Check sheet for the modelled part. Datum: model origin and axes. Units: mm. A direction names the side the tool comes from. Coordinates: 2 decimals unless noted, no trailing zeros. Loops run counter-clockwise (first coordinate to the right, second up) from the corner with the lowest first, then second, coordinate; pieces in that order, holes last.
Autodesk Inventor part; units mm, degrees
ref_plane "YZ Plane" through (0, 0, 0) normal (1, 0, 0) x (0, 1, 0)
ref_plane "XZ Plane" through (0, 0, 0) normal (0, 1, 0) x (-1, 0, 0)
ref_plane "XY Plane" through (0, 0, 0) normal (0, 0, 1) x (1, 0, 0)
sketch "Sketch1" plane through (0, 0, 0) normal (0, 1, 0) x (-1, 0, 0)
  circle A0 centre (0, 0) radius 105
  dimension "d0" = 210
extrude "Extrusion1" add sketch "Sketch1" along normal blind 10
sketch "Sketch2" plane through (0, 10, 0) normal (0, 1, 0) x (1, 0, 0)
  line L0 (-79.8594, -68.6516) -> (79.5179, -68.6516)
  line L1 (0, 0) -> (0, -80)
  line L2 (0, -80) -> (0, -60)
  line L3 (0, -60) -> (17.5, -60)
  line L4 (0, -60) -> (-17.5, -60)
  circle A0 centre (-17.5, -60) radius 2.5
  circle A1 centre (0, -60) radius 2.5
  circle A2 centre (17.5, -60) radius 2.5
  dimension "d4" = 80
  dimension "d5" = 20
  dimension "d6" = 17.5
  dimension "d7" = 17.5
  dimension "d8" = 5
  dimension "d9" = 5
  dimension "d10" = 5
extrude "Extrusion2" cut sketch "Sketch2" against normal blind 10
sketch "Sketch3" plane through (0, 10, 0) normal (0, 1, 0) x (1, 0, 0)
  circle A0 centre (0, 0) radius 2.5
  dimension "d13" = 5
extrude "Extrusion3" cut sketch "Sketch3" against normal blind 10
sketch "Sketch4" plane through (0, 10, 0) normal (0, 1, 0) x (1, 0, 0)
  circle A0 centre (0, 0) radius 2.5
  line L0 (0, 0) -> (0, 80)
  line L1 (-15, 80) -> (-15, 65)
  line L2 (-15, 65) -> (15, 65)
  line L3 (15, 65) -> (15, 95)
  line L4 (15, 95) -> (-15, 95)
  line L5 (-15, 95) -> (-15, 80)
  line L6 (0, 80) -> (-7.5, 80)
  line L7 (-7.5, 80) -> (7.5, 80)
  line L8 (7.5, 80) -> (7.5, 95)
  line L9 (7.5, 80) -> (7.5, 65)
  line L10 (-7.5, 80) -> (-7.5, 95)
  line L11 (-7.5, 80) -> (-7.5, 65)
  dimension "d20" = 15
  dimension "d21" = 15
  dimension "d22" = 30
  dimension "d23" = 30
  dimension "d24" = 7.5
  dimension "d25" = 15
extrude "Extrusion4" add sketch "Sketch4" along normal blind 30 contours L2 L11 L6 L0 | L0 L7 L9 L2 | L6 L10 L4 L8 L7
sketch "Sketch5" plane through (7.5, 10, -65) normal (1, 0, 0) x (0, 0, -1)
  line L0 (40, 0) -> (-170, 0)
  line L1 (40, 0) -> (15, 0)
  line L2 (15, 0) -> (15, 15)
  circle A0 centre (15, 15) radius 7.5
  line L3 (30, 0) -> (30, 30)
  arc A1 (30, 15) -> (0, 15) centre (15, 15) ccw
  line L4 (15, 15) -> (0, 15) construction
  line L5 (15, 15) -> (30, 15) construction
  line L6 (0, 0) -> (0, 30)
  line L7 (0, 15) -> (0, 30)
  line L8 (0, 30) -> (30, 30)
  line L9 (0, 30) -> (30, 30)
  line L10 (30, 30) -> (30, 15)
  point P0 (-65, -10)
  point P1 (15, 30)
  dimension "d28" = 25
  dimension "d29" = 15
  dimension "d30" = 15
  dimension "d31" = 180
extrude "Extrusion5" cut sketch "Sketch5" against normal blind 30 contours A1 L8 L3 | A1 L6 L8 | A0
sketch "Sketch6" plane through (7.5, 10, -65) normal (1, 0, 0) x (0, 0, -1)
  circle A0 centre (15, 15) radius 7.5
  circle A1 centre (15, 15) radius 5
  circle A2 centre (15, 15) radius 7.5
  point P0 (-65, -10)
  dimension "d34" = 10
extrude "Extrusion6" add sketch "Sketch6" against normal blind 15
sketch "Sketch7" plane through (7.5, 10, -65) normal (1, 0, 0) x (0, 0, -1)
  line L0 (0, 0) -> (30, 0)
  line L1 (0, 0) -> (30, 0)
  line L2 (30, 0) -> (30, 34.6991)
  line L3 (30, 34.6991) -> (0, 34.6991)
  line L4 (0, 34.6991) -> (0, 0)
  point P0 (-65, -10)
extrude "Extrusion7" cut sketch "Sketch7" against normal blind 15
sketch "Sketch8" plane through (0, 10, 0) normal (0, 1, 0) x (1, 0, 0)
  circle A0 centre (0, 0) radius 2.5
  line L0 (0, 0) -> (0, 100)
  line L1 (0, 100) -> (-10, 100)
  line L2 (-10, 100) -> (-20, 100)
  line L3 (-20, 100) -> (-20, 65)
  line L4 (-20, 65) -> (-10, 65)
  line L5 (-10, 65) -> (-10, 100)
  line L6 (0, 100) -> (10, 100)
  line L7 (10, 100) -> (20, 100)
  line L8 (20, 100) -> (20, 65)
  line L9 (20, 65) -> (10, 65)
  line L10 (10, 65) -> (10, 100)
  dimension "d42" = 100
  dimension "d43" = 10
  dimension "d44" = 10
  dimension "d45" = 35
  dimension "d46" = 10
  dimension "d47" = 10
  dimension "d48" = 35
extrude "Extrusion8" add sketch "Sketch8" along normal blind 35 contours L5 L4 L3 L2 | L7 L8 L9 L10
thicken "Thicken1" operation add thickness 5 both sides no extend neighbours yes toward (0, 1, 0) faces at (13.3333, 45, -88.3333)
thicken "Thicken2" operation add thickness 5 both sides no extend neighbours yes toward (0, 1, 0) faces at (-16.6667, 45, -88.3333)
sketch "Sketch10" plane through (20, 10, -65) normal (1, 0, 0) x (0, 0, -1)
  line L0 (0, 0) -> (35, 0)
  line L1 (0, 0) -> (17.5, 0)
  line L2 (17.5, 0) -> (17.5, 22.5)
  circle A0 centre (17.5, 22.5) radius 12.5
  circle A1 centre (17.5, 22.5) radius 17.5
  line L3 (35, 0) -> (35, 40)
  line L4 (0, 0) -> (0, 40)
  line L5 (0, 22.5) -> (0, 40)
  line L6 (35, 40) -> (0, 40)
  line L7 (0, 40) -> (35, 40)
  line L8 (35, 40) -> (35, 22.5)
  point P0 (-65, -10)
  point P1 (17.5, 40)
  dimension "d60" = 22.5
  dimension "d61" = 25
extrude "Extrusion9" cut sketch "Sketch10" against normal blind 40 contours L4 L6 A1 | L6 L3 A1 | A0
sketch "Sketch11" plane through (20, 10, -65) normal (1, 0, 0) x (0, 0, -1)
  line L0 (40, 0) -> (-170, 0)
  line L1 (35.2175, 0) -> (0.2175, 0)
  line L2 (0.2175, 0) -> (-34.7825, 0)
  line L3 (0.2175, 0) -> (40.2175, 0)
  circle A0 centre (40.2175, 17.5) radius 12.5
  circle A1 centre (40.2175, 17.5) radius 17.5
  line L4 (-34.7825, 0) -> (32.4725, 33.1928)
  point P0 (-65, -10)
  dimension "d73" = 35
  dimension "d74" = 35
  dimension "d75" = 40
  dimension "d78" = 35
sketch "Sketch12" plane through (-20, 10, -100) normal (-1, 0, 0) x (0, 0, 1)
  line L0 (205, 0) -> (-5, 0)
  line L1 (37.401, 0) -> (37.401, 45.2729)
  line L2 (37.401, 45.2729) -> (-3.1543, 48.8051)
  line L3 (-3.1543, 48.8051) -> (-3.1543, 0)
  line L4 (37.401, 0) -> (-3.1543, 0)
  point P0 (100, -10)
extrude "Extrusion10" cut sketch "Sketch12" against normal blind 40
extrude "Extrusion11" add sketch "Sketch11" against normal blind 40
sketch "Sketch13" plane through (0, 0, 0) normal (0, 0, 1) x (1, 0, 0)
  line L0 (105, 10) -> (-105, 10)
  line L1 (0, 10) -> (10, 10)
  line L2 (10, 10) -> (10, 48.8421)
  line L3 (20, 43.1928) -> (-20, 43.1928)
  line L4 (10, 48.8421) -> (-10, 48.8421)
  line L5 (-10, 48.8421) -> (-10, 10)
  line L6 (-10, 10) -> (10, 10)
  point P0 (0, 0)
  point P1 (-20, 10)
  point P2 (20, 10)
  dimension "d83" = 10
  dimension "d84" = 20
extrude "Extrusion12" cut sketch "Sketch13" against normal blind 150
sketch "Sketch14" plane through (20, 10, -65) normal (1, 0, 0) x (0, 0, -1)
  line L0 (38.0776, 0) -> (-34.7825, 0)
  line L1 (-34.7825, 0) -> (42.8397, 49.7383)
  line L2 (42.8397, 49.7383) -> (77.8644, 0)
  line L3 (77.8644, 0) -> (-34.7825, 0)
  point P0 (-65, -10)
extrude "Extrusion13" cut sketch "Sketch14" against normal blind 150
sketch "Sketch15" plane through (0, 10, 0) normal (0, 1, 0) x (1, 0, 0)
  circle A0 centre (0, 0) radius 2.5
  line L0 (0, 0) -> (0, 100)
  line L1 (0, 100) -> (-20, 100)
  line L2 (-20, 100) -> (-20, 65)
  line L3 (-20, 65) -> (-10, 65)
  line L4 (-10, 65) -> (-10, 100)
  line L5 (-10, 65) -> (10, 65)
  line L6 (10, 65) -> (20, 65)
  line L7 (20, 65) -> (20, 100)
  line L8 (20, 100) -> (10, 100)
  line L9 (10, 100) -> (10, 65)
  dimension "d89" = 100
  dimension "d90" = 20
  dimension "d91" = 35
  dimension "d92" = 10
  dimension "d93" = 20
  dimension "d94" = 10
  dimension "d95" = 35
  dimension "d96" = 10
extrude "Extrusion14" add sketch "Sketch15" along normal blind 40 contours L3 L2 L1 L4 | L9 L8 L7 L6
sketch "Sketch16" plane through (20, 10, -65) normal (1, 0, 0) x (0, 0, -1)
  line L0 (0, 40) -> (35, 40)
  line L1 (17.5, 40) -> (17.5, 22.5)
  circle A0 centre (17.5, 22.5) radius 12.5
  circle A1 centre (17.5, 22.5) radius 17.5
  line L2 (35, 0) -> (35, 40)
  line L3 (0, 0) -> (0, 40)
  line L4 (0, 22.5) -> (0, 40)
  line L5 (0, 40) -> (35, 40)
  line L6 (35, 40) -> (35, 22.5)
  point P0 (-65, -10)
  dimension "d99" = 17.5
  dimension "d100" = 25
extrude "Extrusion15" cut sketch "Sketch16" against normal blind 40 contours L0 A1 L3 | L0 L2 A1 | A0
properties part number "Base do telescópio"
1) Mould release check, pull along Y, two halves, no side actions. Record for faces 4 (the cylindrical face through (-14.93, 49.996, -82.885)), 5 (the cylindrical face through (-14.93, 27.712, -94.047)), 6 (the flat face through (-15, 21, -100)): +Y half, -Y half, draft (parallel to the pull), parting line (faces both ways), or undercut.
Answer sheet:
face 4: +Y half
face 5: undercut
face 6: draft
2) Section check D-D on y = 29.5. Enter the section's corners in (x, z).
Answer sheet:
outline: (-20, -100) - (-10, -100) - (-10, -94.63) - (-20, -94.63) - close; (-20, -70.37) - (-10, -70.37) - (-10, -65) - (-20, -65) - close; (10, -100) - (20, -100) - (20, -94.63) - (10, -94.63) - close; (10, -70.37) - (20, -70.37) - (20, -65) - (10, -65) - close
3) Scan lines: line 1 (Z direction, x = 0, y = 5.75); line 2 (X direction, y = 4, z = 0); line 3 (X direction, y = 2, z = 60). Record each from-to range of solid material in increasing order.
Answer sheet:
line 1: z = -105 to -2.5, 2.5 to 57.5, 62.5 to 105
line 2: x = -105 to -2.5, 2.5 to 105
line 3: x = -86.17 to -20, -15 to -2.5, 2.5 to 15, 20 to 86.17
4) Depth check by flat-ended pin: pin 1 (11 mm diameter, centred on x = -12.5, y = 24.5, fed in from -Z); pin 2 (8 mm diameter, centred on x = 13.5, y = 17.5, fed in from +Z); pin 3 (4.5 mm diameter, centred on x = 17.5, z = 60, fed in from -Y); pin 4 (1 mm diameter, centred on x = -6, z = -48, fed in from +Y). Enter the tip coordinate at first touch or a pass-through.
Answer sheet:
pin 1: stops at z = -100
pin 2: stops at z = -65
pin 3: passes through
pin 4: stops at y = 10
5) Set-up check for faces 1 (the flat face through (10, 21, -75)), 2 (the flat face through (-15, 21, -65)), 3 (the flat face through (-20, 21, -75)): record each of +Z, -Z, +X, -X, +Y, -Y from which the full face is reachable in a straight line by a thin tool's end or side.
Answer sheet:
face 1: +Z, -Z, +Y
face 2: +Z, +X, -X, +Y
face 3: +Z, -Z, -X, +Y
6) Section check C-C on z = -82.5. Enter the section's corners in (x, y).
Answer sheet:
outline: (-64.95, 0) - (64.95, 0) - (64.95, 10) - (20, 10) - (20, 20) - (10, 20) - (10, 10) - (-10, 10) - (-10, 20) - (-20, 20) - (-20, 10) - (-64.95, 10) - close; (-20, 45) - (-10, 45) - (-10, 50) - (-20, 50) - close; (10, 45) - (20, 45) - (20, 50) - (10, 50) - close
7) Section check B-B on y = 15. Enter the section's corners in (x, z), plus the area to 3 significant figures.
Answer sheet:
outline: (-20, -100) - (-10, -100) - (-10, -65) - (-20, -65) - close; (10, -100) - (20, -100) - (20, -65) - (10, -65) - close
area: 700 mm2
8) Section check A-A on x = 0. Enter the section's corners in (y, z), plus the area to 3 significant figures.
Answer sheet:
outline: (0, -105) - (10, -105) - (10, -2.5) - (0, -2.5) - close; (0, 2.5) - (10, 2.5) - (10, 57.5) - (0, 57.5) - close; (0, 62.5) - (10, 62.5) - (10, 105) - (0, 105) - close
area: 2,000 mm2
